```python
from build123d import *

# Parameters (mm, degrees)
F0_W     = 15.7734
F0_H     = 15.7734
F1_DEPTH = 9.5758
F2_R     = 2.4511
F3_DEPTH = 1.8034
F5_W     = 13.1826
F5_H     = 13.1826
F5_R     = 3.1299195118
F6_DEPTH = 8.3566


# Not quite as in the source:
# - a feature names something its author has since deleted; it is built from what else it names


with BuildPart() as f1:
    # F0 (on Top) → F1 (new body)
    with BuildSketch(Plane.XY):
        Rectangle(F0_W, F0_H)
    extrude(amount=F1_DEPTH)

    # F2 (on face) → F3 (join)
    with BuildSketch(Plane.XY.offset(9.5758)):
        with Locations((-4.0386, -3.937)):
            Circle(F2_R)
        with Locations((3.937, -3.937)):
            Circle(F2_R)
        with Locations((3.937, 3.937)):
            Circle(F2_R)
        with Locations((-4.0386, 3.937)):
            Circle(F2_R)
    extrude(amount=F3_DEPTH)

    # F5 (on face) → F6 (cut)
    with BuildSketch(Plane(origin=(0, 0, 0), x_dir=(1, 0, 0), z_dir=(0, 0, -1))):
        Rectangle(F5_W, F5_H)
        Circle(F5_R, mode=Mode.SUBTRACT)
    extrude(amount=-F6_DEPTH, mode=Mode.SUBTRACT)


solid = f1.part
```
Source: CAD feature listing. Evaluate the final solid. Frame: model axes, mm. A direction names the side the tool comes from. Round coordinates to 2 decimals unless told otherwise and drop trailing zeros. Loops run counter-clockwise (first coordinate to the right, second up) from the corner with the lowest first, then second, coordinate; pieces in that order, holes last. Notation, with made-up numbers: M 58.5,76 L 72.5,76 A22 cw 72.5,91 Z; hole C -1,80.25 d8. An arc over 180 degrees is marked long. Put each result on its own line as item: value.
(1) Access query for faces 5 (the face through (-6.591, 0, 4)), 6 (the face through (0, 0, 0)), 7 (the face through (-4.57, 1.544, 10.465)). Directions: +Z, -Z, +X, -X, +Y, -Y. A direction counts if a zero-diameter tool reaches every point of the face in a straight line with its end or side. Return the directions, or none.
Solutions:
face 5: -Z
face 6: -Z, +X, -X, +Y, -Y
face 7: +Z
(2) Section D-D, the plane z = 10. Return loops of the section in (x, y), and give its area (3 significant figures).
Solutions:
outline: C -4.04,-3.94 d4.9; C -4.04,3.94 d4.9; C 3.94,-3.94 d4.9; C 3.94,3.94 d4.9
area: 75.5 mm²
(3) First-contact query: pin 1 (1 mm diameter, centred on x = -3, y = -6, fed in from -Z). Flat tip, straight axial feed; report the tip coordinate or a pass-through.
Solutions:
pin 1: z = 8.36
(4) Ray query, line 1 (Y direction, x = 0, z = 4); line 2 (X direction, y = -4, z = 6.75). Return the intervals inside material, ascending. Write a range as [from, to].
Solutions:
line 1: [-7.89, -6.59], [-3.13, 3.13], [6.59, 7.89]
line 2: [-7.89, -6.59], [6.59, 7.89]
(5) Pull-direction query (Y, two-part tool) for faces 1 (the face through (0, -7.887, 5)), 2 (the face through (4, -4, 11.379)), 3 (the face through (0, -6.591, 4)), 4 (the face through (0, 6.591, 4)); classes: released by +Y, released by -Y, zero draft, split by the parting line, or undercut.
Solutions:
face 1: released by -Y
face 2: zero draft
face 3: undercut
face 4: undercut
(6) Section B-B, the plane y = 0. Return loops of the section in (x, z), and give its area (3 significant figures).
Solutions:
outline: M -7.89,0 L -6.59,0 L -6.59,8.36 L -3.13,8.36 L -3.13,0 L 3.13,0 L 3.13,8.36 L 6.59,8.36 L 6.59,0 L 7.89,0 L 7.89,9.58 L -7.89,9.58 Z
area: 93.2 mm²
(7) Section A-A, the plane z = 3.75. Return loops of the section in (x, y).
Solutions:
outline: M -7.89,-7.89 L 7.89,-7.89 L 7.89,7.89 L -7.89,7.89 Z; C 0,0 d6.26; hole M -6.59,-6.59 L 6.59,-6.59 L 6.59,6.59 L -6.59,6.59 Z
